from build123d import *

# Parameters (mm, degrees)
F0_W     = 73
F0_H     = 59
F1_DEPTH = 5
F2_SIZE  = 25
F4_D     = 3.3
F4_DEPTH = 13.8
F4_TIP   = 0.9914200214
F3_R     = 13.4455987062
F5_DEPTH = 5
F6_W     = 73
F6_H     = 5
F7_DEPTH = 5
F8_W     = 73
F8_H     = 12
F9_DEPTH = 5
F11_D    = 3.2
F12_R    = 5


with BuildPart() as f1:
    # F0 (on Top) → F1 (new body)
    with BuildSketch(Plane.XY):
        Rectangle(F0_W, F0_H)
        with BuildLine():
            Line((-32.5, 13.5), (-32.5, 23.5))
            ThreePointArc((-32.5, 23.5), (-30, 26), (-27.5, 23.5))
            Line((-27.5, 23.5), (-27.5, 13.5))
            ThreePointArc((-27.5, 13.5), (-30, 11), (-32.5, 13.5))
        make_face(mode=Mode.SUBTRACT)
        with BuildLine():
            Line((27.5, 13.5), (27.5, 23.5))
            ThreePointArc((27.5, 23.5), (30, 26), (32.5, 23.5))
            Line((32.5, 23.5), (32.5, 13.5))
            ThreePointArc((32.5, 13.5), (30, 11), (27.5, 13.5))
        make_face(mode=Mode.SUBTRACT)
    extrude(amount=F1_DEPTH)

    # F2
    f2_edges = [f1.edges().sort_by_distance(p)[0] for p in [
        (-36.5, -29.5, 2.5),
        (36.5, -29.5, 2.5),
    ]]
    chamfer(f2_edges, length=F2_SIZE)

    # F4
    with Locations(Plane.XY.offset(5)):
        with Locations((-21.9203102168, -2.5796897832), (0, -24.5), (21.9203102168, -2.5796897832)):
            Hole(F4_D / 2, depth=F4_DEPTH)
            with Locations((0, 0, -(F4_DEPTH + F4_TIP / 2))):  # 118° drill point
                Cone(0, F4_D / 2, F4_TIP, mode=Mode.SUBTRACT)

    # F3 (on face) → F5 (cut, through all)
    with BuildSketch(Plane.XY.offset(5)):
        with Locations((0, -2.5796897832)):
            Circle(F3_R)
    extrude(amount=-F5_DEPTH, mode=Mode.SUBTRACT)

    # F6 (on face) → F7 (join)
    with BuildSketch(Plane(origin=(0, 29.5, 0), x_dir=(-1, 0, 0), z_dir=(0, 1, 0))):
        with Locations((0, 2.5)):
            Rectangle(F6_W, F6_H)
    extrude(amount=F7_DEPTH)

    # F8 (on face) → F9 (join)
    with BuildSketch(Plane(origin=(0, 34.5, 0), x_dir=(-1, 0, 0), z_dir=(0, 1, 0))):
        with Locations((0, 6)):
            Rectangle(F8_W, F8_H)
    extrude(amount=F9_DEPTH)

    # F11 (through all)
    with Locations(Plane(origin=(0, 39.5, 0), x_dir=(-1, 0, 0), z_dir=(0, 1, 0))):
        with Locations((-31.5, 8), (31.5, 8)):
            Hole(F11_D / 2)

    # F12
    f12_edges = [f1.edges().sort_by_distance(p)[0] for p in [
        (36.5, -4.5, 2.5),
        (11.5, -29.5, 2.5),
        (-11.5, -29.5, 2.5),
        (-36.5, -4.5, 2.5),
    ]]
    fillet(f12_edges, radius=F12_R)


solid = f1.part
Could you check a few things on this model? Use its own coordinates, in mm. A direction names the side the tool comes from. Coordinates: 2 decimals unless noted, no trailing zeros. Write each loop counter-clockwise with the first axis right and the second up, starting at its lowest first coordinate (ties: lowest second). Pieces come first, ordered by that corner, then holes. Notation, with made-up numbers: (50, 32.25) - (54, 32.25) arc R13 ccw to (54, 44.25) - close; hole circle Ø3 at (45.5, -29). An arc over 180 degrees is marked (long way). Put each result on its own line as item: value. Start each with the question number.
Q1. I want a section at B-B on z = 8. Write out the boundary of the cut face in (x, y), plus the area to 3 significant figures.
Q2. I want a section at D-D on y = 8. Write out the boundary of the cut face in (x, z), plus the area to 3 significant figures.
Q3. Thinking about a two-plate mould opening in Y: for faces 1 (the cylindrical face through (30, 11, 2)), 2 (the cylindrical face through (-11.37, -29.11, 2.54)), 3 (the flat face through (36.5, 18, 3)), 4 (the flat face through (27.5, 18, 2)), which applies, pulls with the +Y half, pulls with the -Y half, needs draft (parallel to the pull), parting line crosses it, or undercut?
Q4. I want a section at A-A on x = 0. Write out the boundary of the cut face in (y, z), plus the area to 3 significant figures.
Q5. Which directions (+Z, -Z, +X, -X, +Y, -Y) give clear straight access to the entire face, cutting with the end or side of a thin tool? Please do faces 5 (the cylindrical face through (36.13, -4.32, 2.54)), 6 (the flat face through (1, 34.5, 9)), 7 (the cylindrical face through (-30, 26, 2)).
Q6. I'm going to push flat-ended pins straight in: P1, Ø12, axis at x = -14.5, y = 25, coming from the +Z side; P2, Ø3, axis at x = 6, y = 11, coming from the -Z side; P3, Ø3.5, axis at x = 0, z = 8, coming from the -Y side. Where does each tip first touch, or does it pass through?
Q7. I want a section at C-C on y = 20.5. Write out the boundary of the cut face in (x, z), plus the area to 3 significant figures.
Q8. Please list where these lines run through material, in increasing order: L1, parallel to Y at x = 0, z = 3.4; L2, parallel to Z at x = 31.5, y = 35.75; L3, parallel to Z at x = -27.5, y = -10.5.
Checks:
1. outline: (-36.5, 34.5) - (-33.1, 34.5) - (-33.1, 39.5) - (-36.5, 39.5) - close; (-29.9, 34.5) - (29.9, 34.5) - (29.9, 39.5) - (-29.9, 39.5) - close; (33.1, 34.5) - (36.5, 34.5) - (36.5, 39.5) - (33.1, 39.5) - close
1. area: 333 mm²
2. outline: (-36.5, 0) - (-8.3, 0) - (-8.3, 5) - (-36.5, 5) - close; (8.3, 0) - (36.5, 0) - (36.5, 5) - (8.3, 5) - close
2. area: 282 mm²
3. face 1: undercut
3. face 2: pulls with the -Y half
3. face 3: needs draft
3. face 4: undercut
4. outline: (-29.5, 0) - (-26.15, 0) - (-26.15, 5) - (-29.5, 5) - close; (-22.85, 0) - (-16.03, 0) - (-16.03, 5) - (-22.85, 5) - close; (10.87, 0) - (39.5, 0) - (39.5, 12) - (34.5, 12) - (34.5, 5) - (10.87, 5) - close
4. area: 229 mm²
5. face 5: +Z, -Z, +X, -Y
5. face 6: +Z, +X, -X, -Y
5. face 7: +Z, -Z
6. P1: z = 5
6. P2: z = 0
6. P3: y = 34.5
7. outline: (-36.5, 0) - (-32.5, 0) - (-32.5, 5) - (-36.5, 5) - close; (-27.5, 0) - (27.5, 0) - (27.5, 5) - (-27.5, 5) - close; (32.5, 0) - (36.5, 0) - (36.5, 5) - (32.5, 5) - close
7. area: 315 mm²
8. L1: -29.5 to -26.15, -22.85 to -16.03, 10.87 to 39.5
8. L2: 0 to 6.4, 9.6 to 12
8. L3: 0 to 5
